Source: CAD feature listing. Evaluate the final solid. Frame: model axes, mm. Give positions to 0.01 mm unless a question says otherwise; leave off trailing zeros. Loops run counter-clockwise (first coordinate to the right, second up) from the corner with the lowest first, then second, coordinate; pieces in that order, holes last. Notation, with made-up numbers: (4, 17) -> (50, 17) arc R18 ccw to (50, 34) -> close; hole circle Ø1 at (6.25, 77.5). An arc over 180 degrees is marked (long way). Answer as a JSON object with one key per item and string values. Group by question number.
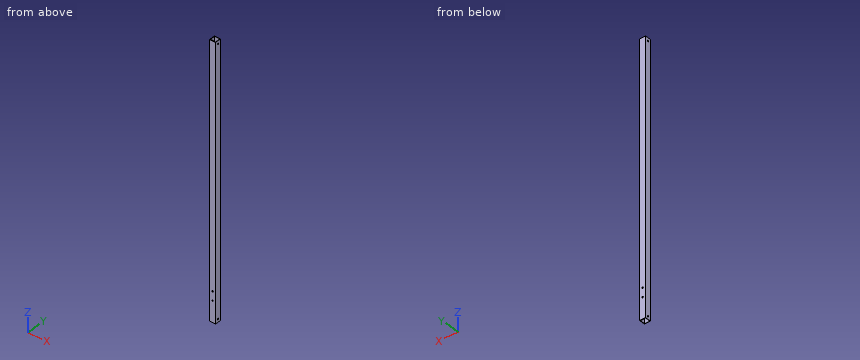
Autodesk Inventor part; units mm, degrees
ref_plane "YZ Plane" through (0, 0, 0) normal (1, 0, 0) x (0, 1, 0)
ref_plane "XZ Plane" through (0, 0, 0) normal (0, 1, 0) x (-1, 0, 0)
ref_plane "XY Plane" through (0, 0, 0) normal (0, 0, 1) x (1, 0, 0)
sketch "Sketch1" plane through (0, 0, 0) normal (0, 0, 1) x (1, 0, 0)
  line L0 (0, 0) -> (25.4, 0)
  line L1 (25.4, 0) -> (25.4, 25.4)
  line L2 (25.4, 25.4) -> (0, 25.4)
  line L3 (0, 25.4) -> (0, 0)
  line L4 (1.5875, 23.8125) -> (23.8125, 23.8125)
  line L5 (23.8125, 23.8125) -> (23.8125, 1.5875)
  line L6 (23.8125, 1.5875) -> (1.5875, 1.5875)
  line L7 (1.5875, 1.5875) -> (1.5875, 23.8125)
  dimension "d0" = 25.4
  dimension "d1" = 25.4
  dimension "d2" = 1.5875
extrude "Extrusion1" add sketch "Sketch1" against normal blind 1143
sketch "Sketch2" plane through (25.4, 0, 0) normal (1, 0, 0) x (0, 0, -1)
  line L0 (1143, 0) -> (1143, 25.4)
  line L1 (0, 0) -> (0, 25.4)
  point P0 (12.7, 12.7)
  point P1 (1130.3, 12.7)
  dimension "d5" = 12.7
  dimension "d6" = 12.7
hole "Hole1" at (25.4, 12.7, -12.7) at (25.4, 12.7, -1130.3) direction (-1, 0, 0) diameter 6.35 depth 25.4 tip angle 118
sketch "Sketch3" plane through (0, 25.4, 0) normal (0, 1, 0) x (1, 0, 0)
  line L0 (25.4, 1143) -> (0, 1143)
  point P0 (12.7, 1016)
  point P1 (12.7, 1054.1)
  dimension "d14" = 38.1
  dimension "d23" = 88.9
hole "Hole2" at (12.7, 25.4, -1016) at (12.7, 25.4, -1054.1) direction (0, -1, 0) diameter 6.35 depth 25.4 tip angle 118
properties part number "1tube_40"
(1) Section query A-A on z = -181. Return the cut outline in (x, y), plus the area to 3 significant figures.
(2) Material intervals for line 1 (Z direction, x = 12.5, y = 24.75); line 2 (Y direction, x = 0.45, z = -1130.3) (3 decimals); line 3 (Z direction, x = 0.45, y = 12.7) (3 decimals), sorted ascending. Write a range as from..to.
(3) First-contact query: pin 1 (5.5 mm diameter, centred on x = 12.7, z = -1054.1, fed in from +Y); pin 2 (8.5 mm diameter, centred on y = 12.7, z = -12.7, fed in from -X). Flat tips, straight axial feed; report the tip coordinate or a pass-through.
Result:
{
 "1": {"outline": "(0, 0) -> (25.4, 0) -> (25.4, 25.4) -> (0, 25.4) -> close; hole (1.59, 1.59) -> (23.81, 1.59) -> (23.81, 23.81) -> (1.59, 23.81) -> close", "area": "151 mm²"},
 "2": {"line 1": "-1143..-1057.27, -1050.93..-1019.17, -1012.83..0", "line 2": "0..9.525, 15.875..25.4", "line 3": "-1143..-1133.475, -1127.125..-15.875, -9.525..0"},
 "3": {"pin 1": "through", "pin 2": "x = 0"}
}
